Read the model definition and answer for the solid it produces. Units are mm, in the model's axes. Round coordinates to 2 decimals unless told otherwise and drop trailing zeros. Answer as a JSON object with one key per item and string values. Group by question number.
Q1. Given pin 1 Ø0.6 at (y, z) = (1, 25) entering from +X; pin 2 Ø0.8 at (y, z) = (0.5, -33.5) entering from -X; pin 3 Ø0.8 at (x, y) = (21, 2.5) entering from +Z; pin 4 Ø0.5 at (y, z) = (2.5, 16) entering from -X, each flat-ended and moving along its own axis, determine where each tip first touches the part or whether it passes through.
Q2. Consider line 1 (Z direction, x = 32, y = 0.4); line 2 (Z direction, x = -21.5, y = 0.85); line 3 (X direction, y = 2.1, z = 65). Determine where each line is inside the solid, lowest interval first.
Q3. A cutting plane is placed at B-B on x = -20. Count the separate pieces of the cut face and the enclosed holes in it, and give its area (3 significant figures).
```python
from build123d import *

# Parameters (mm, degrees)
SKETCH1_W           = 80
SKETCH1_H           = 150
BOSS_EXTRUDE1_DEPTH = 3
SKETCH2_W           = 66
SKETCH2_H           = 31
CUT_EXTRUDE1_DEPTH  = 3
SKETCH4_R           = 7.5
CUT_EXTRUDE2_DEPTH  = 1
SKETCH5_R           = 6.5
CUT_EXTRUDE3_DEPTH  = 19
SKETCH6_R           = 10
CUT_EXTRUDE4_DEPTH  = 1
SKETCH8_R           = 9
CUT_EXTRUDE5_DEPTH  = 86.023526156
SKETCH9_W           = 7
SKETCH9_H           = 7
CUT_EXTRUDE6_DEPTH  = 1
SKETCH12_W          = 5
SKETCH12_H          = 5
CUT_EXTRUDE7_DEPTH  = 86.023526156
FILLET1_R           = 3
FILLET2_R           = 2
SKETCH15_W          = 7
SKETCH15_H          = 7
CUT_EXTRUDE9_DEPTH  = 1
SKETCH16_W          = 5
SKETCH16_H          = 5
CUT_EXTRUDE10_DEPTH = 86.023526156


with BuildPart() as part:
    # Sketch1 → Boss-Extrude1 (new body)
    with BuildSketch(Plane(origin=(0, 0, 0), x_dir=(1, 0, 0), z_dir=(0, 1, 0))):
        Rectangle(SKETCH1_W, SKETCH1_H)
    extrude(amount=BOSS_EXTRUDE1_DEPTH)

    # Sketch2 → Cut-Extrude1 (cut)
    with BuildSketch(Plane(origin=(0, 3, 0), x_dir=(1, 0, 0), z_dir=(0, 1, 0))):
        with Locations((0, 29.5)):
            Rectangle(SKETCH2_W, SKETCH2_H)
    extrude(amount=-CUT_EXTRUDE1_DEPTH, mode=Mode.SUBTRACT)

    # Sketch4 → Cut-Extrude2 (cut)
    with BuildSketch(Plane(origin=(0, 3, 0), x_dir=(1, 0, 0), z_dir=(0, 1, 0))):
        with Locations(Location((0, 60, 0), (0, 0, 270))):
            Circle(SKETCH4_R)
    extrude(amount=-CUT_EXTRUDE2_DEPTH, mode=Mode.SUBTRACT)

    # Sketch5 → Cut-Extrude3 (cut)
    with BuildSketch(Plane(origin=(0, 2, 0), x_dir=(1, 0, 0), z_dir=(0, 1, 0))):
        with Locations(Location((0, 60, 0), (0, 0, 270))):
            Circle(SKETCH5_R)
    extrude(amount=-CUT_EXTRUDE3_DEPTH, mode=Mode.SUBTRACT)

    # Sketch6 → Cut-Extrude4 (cut)
    with BuildSketch(Plane(origin=(0, 3, 0), x_dir=(1, 0, 0), z_dir=(0, 1, 0))):
        with Locations(Location((-20, -16, 0), (0, 0, 270))):
            Circle(SKETCH6_R)
    extrude(amount=-CUT_EXTRUDE4_DEPTH, mode=Mode.SUBTRACT)

    # Sketch8 → Cut-Extrude5 (cut, through all)
    with BuildSketch(Plane(origin=(0, 2, 0), x_dir=(1, 0, 0), z_dir=(0, 1, 0))):
        with Locations(Location((-20, -16, 0), (0, 0, 270))):
            Circle(SKETCH8_R)
    extrude(amount=-CUT_EXTRUDE5_DEPTH, mode=Mode.SUBTRACT)

    # Sketch9 → Cut-Extrude6 (cut)
    with BuildSketch(Plane(origin=(0, 3, 0), x_dir=(1, 0, 0), z_dir=(0, 1, 0))):
        with Locations((20, -6)):
            Rectangle(SKETCH9_W, SKETCH9_H)
        with Locations((20, -26)):
            Rectangle(SKETCH9_W, SKETCH9_H)
        with Locations((10, -16)):
            Rectangle(SKETCH9_W, SKETCH9_H)
        with Locations((30, -16)):
            Rectangle(SKETCH9_W, SKETCH9_H)
    extrude(amount=-CUT_EXTRUDE6_DEPTH, mode=Mode.SUBTRACT)

    # Sketch12 → Cut-Extrude7 (cut, through all)
    with BuildSketch(Plane(origin=(0, 2, 0), x_dir=(1, 0, 0), z_dir=(0, 1, 0))):
        with Locations((20, -6)):
            Rectangle(SKETCH12_W, SKETCH12_H)
        with Locations((10, -16)):
            Rectangle(SKETCH12_W, SKETCH12_H)
        with Locations((30, -16)):
            Rectangle(SKETCH12_W, SKETCH12_H)
        with Locations((20, -26)):
            Rectangle(SKETCH12_W, SKETCH12_H)
    extrude(amount=-CUT_EXTRUDE7_DEPTH, mode=Mode.SUBTRACT)

    # Cut-Extrude8 cone 1 section (through the dimple's axis) → Cut-Extrude8 (revolve, cut)
    with BuildSketch(Plane(origin=(0, 3, 65), x_dir=(0, 0, 1), z_dir=(1, 0, 0))):
        Polygon((0, 0), (1, 0), (0, 3.732050808), align=None)
    revolve(axis=Axis((0, 3, 65), (0, -1, 0)), mode=Mode.SUBTRACT)

    # Cut-Extrude8 cone 2 section (through the dimple's axis) → Cut-Extrude8 cone 2 (revolve, cut)
    with BuildSketch(Plane(origin=(-7.5, 3, 65), x_dir=(0, 0, 1), z_dir=(1, 0, 0))):
        Polygon((0, 0), (1, 0), (0, 3.732050808), align=None)
    revolve(axis=Axis((-7.5, 3, 65), (0, -1, 0)), mode=Mode.SUBTRACT)

    # Cut-Extrude8 cone 3 section (through the dimple's axis) → Cut-Extrude8 cone 3 (revolve, cut)
    with BuildSketch(Plane(origin=(-15, 3, 65), x_dir=(0, 0, 1), z_dir=(1, 0, 0))):
        Polygon((0, 0), (1, 0), (0, 3.732050808), align=None)
    revolve(axis=Axis((-15, 3, 65), (0, -1, 0)), mode=Mode.SUBTRACT)

    # Cut-Extrude8 cone 4 section (through the dimple's axis) → Cut-Extrude8 cone 4 (revolve, cut)
    with BuildSketch(Plane(origin=(7.5, 3, 65), x_dir=(0, 0, 1), z_dir=(1, 0, 0))):
        Polygon((0, 0), (1, 0), (0, 3.732050808), align=None)
    revolve(axis=Axis((7.5, 3, 65), (0, -1, 0)), mode=Mode.SUBTRACT)

    # Cut-Extrude8 cone 5 section (through the dimple's axis) → Cut-Extrude8 cone 5 (revolve, cut)
    with BuildSketch(Plane(origin=(15, 3, 65), x_dir=(0, 0, 1), z_dir=(1, 0, 0))):
        Polygon((0, 0), (1, 0), (0, 3.732050808), align=None)
    revolve(axis=Axis((15, 3, 65), (0, -1, 0)), mode=Mode.SUBTRACT)

    # Fillet1
    fillet1_edges = [part.edges().sort_by_distance(p)[0] for p in [
        (40, 3, 0),
        (0, 3, -75),
        (-40, 3, 0),
        (0, 3, 75),
    ]]
    fillet(fillet1_edges, radius=FILLET1_R - 0.0001)  # a hair under: the kernel refuses the full size

    # Fillet2
    fillet2_edges = [part.edges().sort_by_distance(p)[0] for p in [
        (33, 3, -29.5),
        (0, 3, -45),
        (-33, 3, -29.5),
        (0, 3, -14),
    ]]
    fillet(fillet2_edges, radius=FILLET2_R)

    # Sketch15 → Cut-Extrude9 (cut)
    with BuildSketch(Plane(origin=(0, 3, 0), x_dir=(1, 0, 0), z_dir=(0, 1, 0))):
        with Locations((20, -16)):
            Rectangle(SKETCH15_W, SKETCH15_H)
    extrude(amount=-CUT_EXTRUDE9_DEPTH, mode=Mode.SUBTRACT)

    # Sketch16 → Cut-Extrude10 (cut, through all)
    with BuildSketch(Plane(origin=(0, 2, 0), x_dir=(1, 0, 0), z_dir=(0, 1, 0))):
        with Locations((20, -16)):
            Rectangle(SKETCH16_W, SKETCH16_H)
    extrude(amount=-CUT_EXTRUDE10_DEPTH, mode=Mode.SUBTRACT)


solid = part.part
```
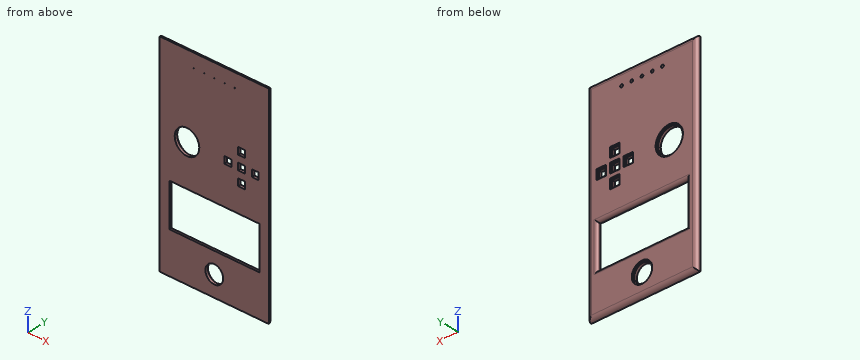
Result set:
{
 "1": {"pin 1": "stops at x = 39.92", "pin 2": "stops at x = -40", "pin 3": "stops at z = 74.14", "pin 4": "stops at x = -38.98"},
 "2": {"line 1": "z = -74.97 to -45, -14 to 13.5, 18.5 to 74.97", "line 2": "z = -74.88 to -45, -14 to 7.13, 24.87 to 74.88", "line 3": "x = -39.14 to -15.76, -14.24 to -8.26, -6.74 to -0.76, 0.76 to 6.74, 8.26 to 14.24, 15.76 to 39.14"},
 "3": {"separate pieces": "3", "enclosed holes": "0", "area": "295 mm²"}
}
